Autodesk Inventor part; units mm, degrees
ref_plane "YZ Plane" through (0, 0, 0) normal (1, 0, 0) x (0, 1, 0)
ref_plane "XZ Plane" through (0, 0, 0) normal (0, 1, 0) x (-1, 0, 0)
ref_plane "XY Plane" through (0, 0, 0) normal (0, 0, 1) x (1, 0, 0)
sketch "Sketch1" plane through (0, 0, 0) normal (0, 0, 1) x (1, 0, 0)
  circle A0 centre (0, 0.0481) radius 3
  circle A1 centre (0, 0.0481) radius 1.5
  circle A2 centre (0, 0.0481) radius 5.5
  arc A3 (2.6218, 17.0122) -> (-2.3779, 17.0481) centre (0.1221, 17.0481) ccw
  line L0 (0.1221, 17.0481) -> (-2.3779, 17.0481) construction
  line L1 (0.1221, 17.0481) -> (2.6221, 17.0481) construction
  line L2 (2.6221, 17.0481) -> (0.1221, 17.0481) construction
  line L3 (-2.3779, 17.0481) -> (-4.4642, 0.6149)
  line L4 (0.1221, 17.0481) -> (0, 0.0481) construction
  line L5 (2.6218, 17.0122) -> (4.4718, 0.5507)
  line L6 (0, 0.0481) -> (-9.4947, 0.1163) construction
  arc A4 (-2.6218, -16.916) -> (2.3779, -16.9519) centre (-0.1221, -16.9519) ccw
  line L7 (-2.6218, -16.916) -> (-4.4718, -0.4544)
  line L8 (2.3779, -16.9519) -> (4.4642, -0.5186)
  arc A5 (-4.4642, 0.6149) -> (-4.4718, -0.4544) centre (0, 0.0481) ccw
  arc A6 (4.4642, -0.5186) -> (4.4718, 0.5507) centre (0, 0.0481) ccw
  circle A7 centre (0, 0.0481) radius 4.5
  dimension "d1" = 3
  dimension "d2" = 6
  dimension "d4" = 11
  dimension "d5" = 5
  dimension "d6" = 17
  dimension "d8" = 16.5652
  dimension "d9" = 16.5652
  dimension "d10" = 97.235
  dimension "d20" = 13.9277
extrude "Extrusion1" add sketch "Sketch1" along normal blind 1.5 contours L5 A7 L3 A2 | A2 L3 A3 L5 | L8 A4 L7 A2 | A2 L7 A7 L8 | A6 A7 A5
extrude "Extrusion2" add sketch "Sketch1" along normal blind 1.5 contours A2 L8 A6 L5 | L5 A7 L3 A2 | A2 L7 A7 L8 | L3 A5 L7 A2 | A6 A7 A5
extrude "Extrusion3" add sketch "Sketch1" against normal blind 3.5 contours A6 A7 A5
extrude "Extrusion4" add sketch "Sketch1" along normal blind 1.5 contours A0
sketch "Sketch2" plane through (0, 0, 1.5) normal (0, 0, 1) x (1, 0, 0)
  circle A0 centre (0, 0.0481) radius 3
  circle A1 centre (0, 10.0481) radius 1.5
  circle A2 centre (0, -9.9519) radius 1.5
  dimension "d25" = 3
  dimension "d26" = 3
  dimension "d29" = 10
  dimension "d30" = 10
extrude "Extrusion5" cut sketch "Sketch2" against normal blind 2 contours A1 | A2
sketch "Sketch3" plane through (0, 0.0481, 0) normal (0, 0, -1) x (-1, 0, 0)
  circle A0 centre (0, 0) radius 1.5
  circle A1 centre (0, 0) radius 3
  point P0 (0, -0.0481)
extrude "Extrusion6" cut sketch "Sketch3" against normal up to next
sketch "Sketch4" plane through (0, 0, 1.5) normal (0, 0, 1) x (1, 0, 0)
  circle A0 centre (0, -9.9519) radius 1.5
  circle A1 centre (0, 10.0481) radius 1.5
  line L0 (2.6218, 17.0122) -> (4.1187, 3.6932)
  arc A2 (2.6218, 17.0122) -> (-2.3779, 17.0481) centre (0.1221, 17.0481) ccw
  line L1 (-4.0659, 3.752) -> (-2.3779, 17.0481)
  line L2 (-2.6218, -16.916) -> (-4.1187, -3.5969)
  arc A3 (-2.6218, -16.916) -> (2.3779, -16.9519) centre (-0.1221, -16.9519) ccw
  line L3 (4.0659, -3.6557) -> (2.3779, -16.9519)
  line L4 (0.1221, 17.0481) -> (0, 10.0481) construction
  line L5 (0, -9.9519) -> (-0.1221, -16.9519) construction
  arc A4 (-2.9596, -13.91) -> (2.7589, -13.9512) centre (0, 0) ccw
  arc A5 (2.9707, 13.9077) -> (-2.7714, 13.9487) centre (0, 0) ccw
extrude "Extrusion7" cut sketch "Sketch4" against normal up to next contours L0 A5 L1 A2 | L2 A4 L3 A3
fillet "Fillet1" radius 2 4 edges at (2.7589, -13.9512, 0.75) (-2.9596, -13.91, 0.75) (2.9707, 13.9077, 0.75) (-2.7714, 13.9487, 0.75)
properties part number "acople para eje falso"
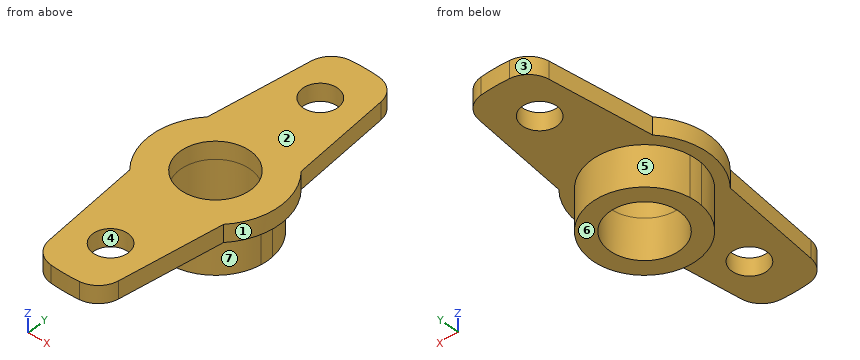
Source: CAD feature listing. Evaluate the final solid. Frame: model axes, mm. Face numbers are marked on the shaded views. A direction names the side the tool comes from. Give positions to 0.01 mm unless a question says otherwise; leave off trailing zeros. Loops run counter-clockwise (first coordinate to the right, second up) from the corner with the lowest first, then second, coordinate; pieces in that order, holes last. Notation, with made-up numbers: (62.25, -15) -> (74.25, -15) arc R26 cw to (74.25, 12) -> close; hole circle Ø6 at (-16.5, 19). An arc over 180 degrees is marked (long way). Use a Markdown table: item, result. Add a question column.
(1) Pull-direction query (X, two-part tool) for the marked faces 1, 2, 3 and 4; classes: +X half, -X half, draft (parallel to the pull), parting line (faces both ways), or undercut.
(2) First-contact query: pin 1 Ø2 at (x, y) = (4.5, 6.5) entering from -Z; pin 2 Ø1.5 at (x, z) = (-1, -1) entering from +Y; pin 3 Ø1.5 at (x, z) = (-4, -2) entering from -Y. Flat tips, straight axial feed; report the tip coordinate or a pass-through.
(3) Section query B-B (y = -2.25). Output: boundary loops of the cut face in (x, z).
(4) Section query A-A (x = 0). Output: boundary loops of the cut face in (y, z), then the cut area to 3 significant figures.
(5) Access query for the marked faces 5, 6 and 7. Directions: +Z, -Z, +X, -X, +Y, -Y. A direction counts if a zero-diameter tool reaches every point of the face in a straight line with its end or side. Return the directions, or none.
(6) Section query C-C (z = -2.8). Output: boundary loops of the cut face in (x, y), then the cut area to 3 significant figures.
(7) Section query D-D (x = 2). Output: boundary loops of the cut face in (y, z), then the cut area to 3 significant figures.
(8) Ray query, line 1 (Y direction, x = 0, z = 0.4); line 2 (X direction, y = -0.5, z = -2.45); line 3 (Y direction, x = 0, z = -0.85). Return the intervals inside material, ascending.
Checked values:
| question | item | result |
|---|---|---|
| 1 | face 1 | +X half |
| 1 | face 2 | draft |
| 1 | face 3 | -X half |
| 1 | face 4 | undercut |
| 2 | pin 1 | z = 0 |
| 2 | pin 2 | y = 4.54 |
| 2 | pin 3 | y = -3.06 |
| 3 | outline | (-5, 0) -> (-3.87, 0) -> (-3.87, -3.5) -> (-1.93, -3.5) -> (-1.93, 1.5) -> (-5, 1.5) -> close; (1.93, -3.5) -> (3.87, -3.5) -> (3.87, 0) -> (5, 0) -> (5, 1.5) -> (1.93, 1.5) -> close |
| 4 | outline | (-14.22, 0) -> (-11.45, 0) -> (-11.45, 1.5) -> (-14.22, 1.5) -> close; (-8.45, 0) -> (-4.45, 0) -> (-4.45, -3.5) -> (-2.95, -3.5) -> (-2.95, 1.5) -> (-8.45, 1.5) -> close; (3.05, -3.5) -> (4.55, -3.5) -> (4.55, 0) -> (8.55, 0) -> (8.55, 1.5) -> (3.05, 1.5) -> close; (11.55, 0) -> (14.22, 0) -> (14.22, 1.5) -> (11.55, 1.5) -> close |
| 4 | area | 35.2 mm^2 |
| 5 | face 5 | -Z, +Y |
| 5 | face 6 | -Z, +X, -X, +Y, -Y |
| 5 | face 7 | -Z, -Y |
| 6 | outline | (-4.47, -0.45) arc R4.5 ccw to (4.46, -0.52) arc R4.5 ccw to (4.47, 0.55) arc R4.5 ccw to (-4.46, 0.61) arc R4.49 ccw to start; hole circle Ø6 at (0, 0.05) |
| 6 | area | 35.3 mm^2 |
| 7 | outline | (-13.9, 0) -> (-3.98, 0) -> (-3.98, -3.5) -> (-2.19, -3.5) -> (-2.19, 1.5) -> (-13.9, 1.5) -> close; (2.28, -3.5) -> (4.08, -3.5) -> (4.08, 0) -> (13.98, 0) -> (13.98, 1.5) -> (2.28, 1.5) -> close |
| 7 | area | 47.7 mm^2 |
| 8 | line 1 | -14.22 to -11.45, -8.45 to -2.95, 3.05 to 8.55, 11.55 to 14.22 |
| 8 | line 2 | -4.47 to -2.95, 2.95 to 4.47 |
| 8 | line 3 | -4.45 to -2.95, 3.05 to 4.55 |
